Verification items for this drawing (mm, ordinates from the low corner). A direction names the side the tool comes from. Round coordinates to 2 decimals unless told otherwise and drop trailing zeros. Write each loop counter-clockwise with the first axis right and the second up, starting at its lowest first coordinate (ties: lowest second). Pieces come first, ordered by that corner, then holes.
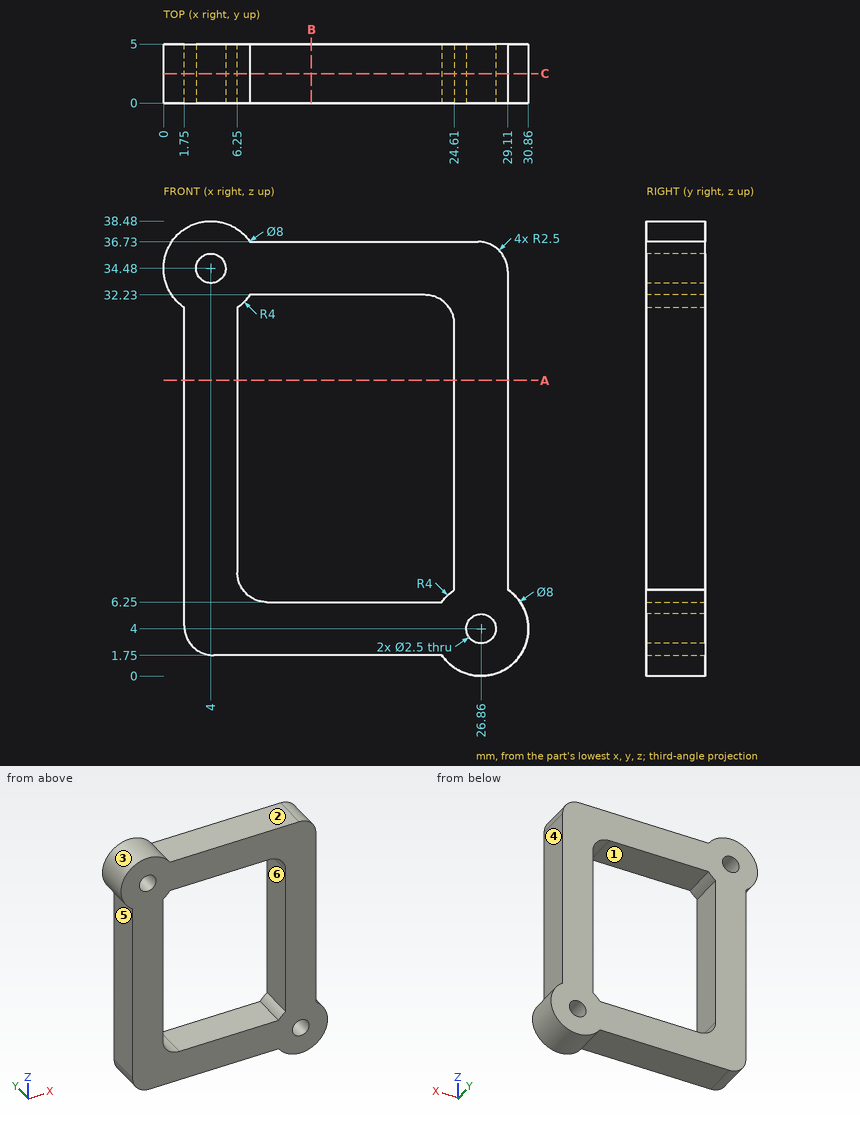
1. Scan lines: line 1 along Z through (x, y) = (11, 1.4); line 2 along X through (y, z) = (1.45, 12); line 3 along X through (y, z) = (1.1, 4). Record each from-to range of solid material in increasing order.
2. Section check C-C (y = 2.5). Record the cut outline in (x, z).
3. Access from +Z, -Z, +X, -X, +Y, -Y to the whole of each face (thin tool, end or side, straight path). Record for the marked faces 4, 5 and 6.
4. Section check B-B (x = 12.5). Record the cut outline in (y, z).
5. Depth check by flat-ended pin: pin 1 Ø2.5 at (y, z) = (2.5, 17) entering from +X; pin 2 Ø3 at (x, z) = (4, 34.48) entering from +Y; pin 3 Ø2 at (x, y) = (13, 4.5) entering from +Z; pin 4 Ø2.5 at (x, y) = (13.5, 1.5) entering from -Z. Enter the tip coordinate at first touch or a pass-through.
6. Section check A-A (z = 25). Record the cut outline in (x, y).
7. Release check for a two-part mould opening along Z. For the marked faces 1, 2 and 3 record: +Z half, -Z half, draft (parallel to the pull), parting line (faces both ways), or undercut.
Results below:
1. line 1: z = 1.75 to 6.25, 32.23 to 36.73
1. line 2: x = 1.75 to 6.25, 24.61 to 29.11
1. line 3: x = 1.76 to 25.61, 28.11 to 30.86
2. outline: (1.75, 4.25) arc R2.5 ccw to (4.25, 1.75) - (23.55, 1.75) arc R4 ccw (long way) to (29.11, 7.31) - (29.11, 34.23) arc R2.5 ccw to (26.61, 36.73) - (7.31, 36.73) arc R4 ccw (long way) to (1.75, 31.17) - close; hole circle Ø2.5 at (4, 34.48); hole (6.25, 8.75) arc R2.5 ccw to (8.75, 6.25) - (23.55, 6.25) arc R4 cw to (24.61, 7.31) - (24.61, 29.73) arc R2.5 ccw to (22.11, 32.23) - (7.31, 32.23) arc R4 cw to (6.25, 31.17) - close; hole circle Ø2.5 at (26.86, 4)
3. face 4: +Z, +X, +Y, -Y
3. face 5: -Z, -X, +Y, -Y
3. face 6: +Y, -Y
4. outline: (0, 1.75) - (5, 1.75) - (5, 6.25) - (0, 6.25) - close; (0, 32.23) - (5, 32.23) - (5, 36.73) - (0, 36.73) - close
5. pin 1: stops at x = 29.11
5. pin 2: stops at y = 5
5. pin 3: stops at z = 36.73
5. pin 4: stops at z = 1.75
6. outline: (1.75, 0) - (6.25, 0) - (6.25, 5) - (1.75, 5) - close; (24.61, 0) - (29.11, 0) - (29.11, 5) - (24.61, 5) - close
7. face 1: undercut
7. face 2: +Z half
7. face 3: parting line
